from build123d import *

# Parameters (mm, degrees)
SKETCH1_W           = 64.5
SKETCH1_H           = 42
BOSS_EXTRUDE1_DEPTH = 3
CUT_EXTRUDE1_REACH  = 79.028
SKETCH2_W           = 29
SKETCH2_H           = 12.5
SKETCH2_H_2         = 12
SKETCH2_W_2         = 9.7
SKETCH2_H_3         = 20
SKETCH5_W           = 64.5
SKETCH5_H           = 2.5
BOSS_EXTRUDE4_DEPTH = 5
CUT_EXTRUDE2_REACH  = 79.131
SKETCH4_R           = 1.25


with BuildPart() as part:
    # Sketch1 → Boss-Extrude1 (new body)
    with BuildSketch(Plane(origin=(0, 0, 0), x_dir=(1, 0, 0), z_dir=(0, 1, 0))):
        with Locations((32.25, 21)):
            Rectangle(SKETCH1_W, SKETCH1_H)
    extrude(amount=BOSS_EXTRUDE1_DEPTH)

    # Sketch2 → Cut-Extrude1 (cut, up to next)
    with BuildSketch(Plane(origin=(0, 3, 0), x_dir=(1, 0, 0), z_dir=(0, 1, 0)), mode=Mode.PRIVATE) as cut_extrude1_sk1:
        with Locations((48, 9.25)):
            Rectangle(SKETCH2_W, SKETCH2_H)
    cut_extrude1_tool1 = extrude(cut_extrude1_sk1.sketch, amount=-CUT_EXTRUDE1_REACH, mode=Mode.PRIVATE) & part.part
    # Sketch2 → Cut-Extrude1 (cut, up to next)
    with BuildSketch(Plane(origin=(0, 3, 0), x_dir=(1, 0, 0), z_dir=(0, 1, 0)), mode=Mode.PRIVATE) as cut_extrude1_sk2:
        with Locations((16.5, 9.5)):
            Rectangle(SKETCH2_W, SKETCH2_H_2)
    cut_extrude1_tool2 = extrude(cut_extrude1_sk2.sketch, amount=-CUT_EXTRUDE1_REACH, mode=Mode.PRIVATE) & part.part
    # Sketch2 → Cut-Extrude1 (cut, up to next)
    with BuildSketch(Plane(origin=(0, 3, 0), x_dir=(1, 0, 0), z_dir=(0, 1, 0)), mode=Mode.PRIVATE) as cut_extrude1_sk3:
        with Locations((6.85, 27.5)):
            Rectangle(SKETCH2_W_2, SKETCH2_H_3)
    cut_extrude1_tool3 = extrude(cut_extrude1_sk3.sketch, amount=-CUT_EXTRUDE1_REACH, mode=Mode.PRIVATE) & part.part
    add(cut_extrude1_tool1.solids().sort_by_distance((48, 3, -9.25))[0], mode=Mode.SUBTRACT)
    add(cut_extrude1_tool2.solids().sort_by_distance((16.5, 3, -9.5))[0], mode=Mode.SUBTRACT)
    add(cut_extrude1_tool3.solids().sort_by_distance((6.85, 3, -27.5))[0], mode=Mode.SUBTRACT)

    # Sketch5 → Boss-Extrude4 (add)
    with BuildSketch(Plane.XZ):
        with Locations((32.25, -1.25)):
            Rectangle(SKETCH5_W, SKETCH5_H)
    extrude(amount=BOSS_EXTRUDE4_DEPTH)

    # Sketch4 → Cut-Extrude2 (cut, up to next)
    with BuildSketch(Plane.XY, mode=Mode.PRIVATE) as cut_extrude2_sk1:
        with Locations((62, -2.5)):
            Circle(SKETCH4_R)
    cut_extrude2_tool1 = extrude(cut_extrude2_sk1.sketch, amount=-CUT_EXTRUDE2_REACH, mode=Mode.PRIVATE) & part.part
    # Sketch4 → Cut-Extrude2 (cut, up to next)
    with BuildSketch(Plane.XY, mode=Mode.PRIVATE) as cut_extrude2_sk2:
        with Locations((6, -2.5)):
            Circle(SKETCH4_R)
    cut_extrude2_tool2 = extrude(cut_extrude2_sk2.sketch, amount=-CUT_EXTRUDE2_REACH, mode=Mode.PRIVATE) & part.part
    # Sketch4 → Cut-Extrude2 (cut, up to next)
    with BuildSketch(Plane.XY, mode=Mode.PRIVATE) as cut_extrude2_sk3:
        with Locations((34, -2.5)):
            Circle(SKETCH4_R)
    cut_extrude2_tool3 = extrude(cut_extrude2_sk3.sketch, amount=-CUT_EXTRUDE2_REACH, mode=Mode.PRIVATE) & part.part
    add(cut_extrude2_tool1.solids().sort_by_distance((62, -2.5, 0))[0], mode=Mode.SUBTRACT)
    add(cut_extrude2_tool2.solids().sort_by_distance((6, -2.5, 0))[0], mode=Mode.SUBTRACT)
    add(cut_extrude2_tool3.solids().sort_by_distance((34, -2.5, 0))[0], mode=Mode.SUBTRACT)


solid = part.part
The listing builds one solid part. Answer for the finished solid, in the listing's coordinates (mm). A direction names the side the tool comes from. Coordinates: 2 decimals unless noted, no trailing zeros. Write each loop counter-clockwise with the first axis right and the second up, starting at its lowest first coordinate (ties: lowest second). Pieces come first, ordered by that corner, then holes. Notation, with made-up numbers: (-13, 15.5) - (4, 15.5) arc R8 ccw to (4, 29.5) - close; hole circle Ø3 at (53.5, 78.25). An arc over 180 degrees is marked (long way). Put each result on its own line as item: value.
1. Determine the mould class of faces 1 (the face through (0, 1, -20)), 2 (the face through (32, -2, -2.5)), 3 (the face through (2, 2, -9)) for opening direction Z: pulls with the +Z half, pulls with the -Z half, needs draft (parallel to the pull), parting line crosses it, or undercut.
Answer sheet:
face 1: needs draft
face 2: pulls with the -Z half
face 3: undercut
2. The part is cut by section C-C on z = -5. Give the vertices of the cut face in (x, y), plus the area to 3 significant figures.
Answer sheet:
outline: (0, 0) - (2, 0) - (2, 3) - (0, 3) - close; (31, 0) - (33.5, 0) - (33.5, 3) - (31, 3) - close; (62.5, 0) - (64.5, 0) - (64.5, 3) - (62.5, 3) - close
area: 19.5 mm^2
3. The part is cut by section B-B on x = 38.5. Give the vertices of the cut face in (y, z), plus the area to 3 significant figures.
Answer sheet:
outline: (-5, -2.5) - (0, -2.5) - (0, -3) - (3, -3) - (3, 0) - (-5, 0) - close; (0, -42) - (3, -42) - (3, -15.5) - (0, -15.5) - close
area: 101 mm^2
4. A tool of negligible diameter and unlimited length cuts with its end or side. For faces 4 (the face through (2, 2, -27)), 5 (the face through (35.19, -2.12, -1.23)), 6 (the face through (39, 0, -27)), from which of +Z, -Z, +X, -X, +Y, -Y can it reach the whole face along a straight path? Write none if from no direction.
Answer sheet:
face 4: +Y, -Y
face 5: +Z, -Z
face 6: -Z, +X, -X, -Y
5. A flat-ended cylindrical pin translates along its axis: pin 1 Ø3 at (y, z) = (1.5, -12) entering from -X. Find the tip coordinate at first contact, or state that the pin passes through.
Answer sheet:
pin 1: stops at x = 0
6. The part is cut by section D-D on x = 6. Give the vertices of the cut face in (y, z), plus the area to 4 significant figures.
Answer sheet:
outline: (-5, -2.5) - (-3.75, -2.5) - (-3.75, 0) - (-5, 0) - close; (-1.25, -2.5) - (0, -2.5) - (0, -3.5) - (3, -3.5) - (3, 0) - (-1.25, 0) - close; (0, -42) - (3, -42) - (3, -37.5) - (0, -37.5) - close; (0, -17.5) - (3, -17.5) - (3, -15.5) - (0, -15.5) - close
area: 36.25 mm^2
7. The part is cut by section A-A on z = -25.5. Give the vertices of the cut face in (x, y), plus the area to 3 significant figures.
Answer sheet:
outline: (0, 0) - (2, 0) - (2, 3) - (0, 3) - close; (11.7, 0) - (64.5, 0) - (64.5, 3) - (11.7, 3) - close
area: 164 mm^2
8. Find the intervals of material crossed by line 1 along Y through (x, z) = (34, -1.3); line 2 along Z through (x, y) = (24.5, 2); line 3 along Z through (x, y) = (40, 1.5), in increasing order. Write a range as from..to.
Answer sheet:
line 1: y = -5..-3.75, -1.25..3
line 2: z = -42..-15.5, -3.5..0
line 3: z = -42..-15.5, -3..0
